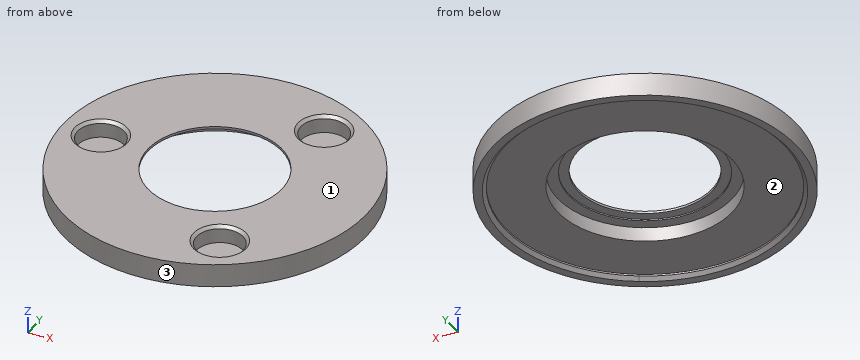
Autodesk Inventor part; units mm, degrees
ref_plane "YZ Plane" through (0, 0, 0) normal (1, 0, 0) x (0, 1, 0)
ref_plane "XZ Plane" through (0, 0, 0) normal (0, 1, 0) x (-1, 0, 0)
ref_plane "XY Plane" through (0, 0, 0) normal (0, 0, 1) x (1, 0, 0)
ref_plane "Arbeitsebene1" through (0, -18.5, -1.048) normal (1, 0, 0) x (0, 0, -1)
sketch "Skizze1" plane through (0, -18.5, -1.048) normal (1, 0, 0) x (0, 0, -1)
  line L0 (-1.65, 12.5) -> (-1.5, 12.5)
  line L1 (-1.5, -12.5) -> (-1.5, 12.5)
  line L2 (-1.65, 12.5) -> (-1.65, -12.5)
  line L3 (8.4324, 0) -> (-3.3304, 0)
  line L4 (-1.6429, 13.1) -> (-1.65, 13.1)
  line L5 (-1.65, 13.1) -> (-1.65, 11.5)
  line L6 (-1.65, 11.5) -> (-2.05, 11.5)
  line L7 (-2.05, 11.5) -> (-2.05, 23.9922)
  line L8 (-2.05, 23.9922) -> (1.05, 23.9922)
  line L9 (1.05, 23.9922) -> (1.05, 14.9922)
  line L10 (1.552, 13.5) -> (-1.048, 13.5) construction
  line L11 (-1.65, 13.1) -> (-1.4, 13.1)
  line L12 (-1.4, 13.1) -> (-1.4, 14.9922)
  line L13 (-1.4, 14.9922) -> (1.05, 14.9922)
  point P0 (-1.048, 18.5)
  dimension "d0" = 0.4
  dimension "d1" = 3.1
  dimension "d2" = 9
  dimension "d3" = 0.6
  dimension "d4" = 0
  dimension "d5" = 1
  dimension "d6" = 0.25
revolve "Umdrehung1" add sketch "Skizze1" angle 360 about axis through (0, -18.5, -9.4804) along (0, 0, 1) contours L2 L6 L7 L8 L9 L13 L12 L11 L4 L5
sketch "Skizze2" plane through (0, -18.5, 1.002) normal (0, 0, -1) x (-1, 0, 0)
  circle A0 centre (0, 0) radius 14.9922
  circle A1 centre (0, 0) radius 23.9922
  line L0 (19.4922, 0) -> (-9.7461, -16.8807) construction
  line L1 (-9.7461, -16.8807) -> (-9.7461, 16.8807) construction
  line L2 (-9.7461, 16.8807) -> (19.4922, 0) construction
  circle A2 centre (19.4922, 0) radius 4
  circle A3 centre (-9.7461, -16.8807) radius 4
  circle A4 centre (-9.7461, 16.8807) radius 4
  point P0 (0, 18.5)
  dimension "d8" = 47.9844
  dimension "d9" = 29.9844
  dimension "d10" = 19.4922
  dimension "d11" = 8
  dimension "d12" = 8
  dimension "d13" = 8
extrude "Extrusion1" cut sketch "Skizze2" along normal blind 3 contours A2 | A3 | A4
chamfer "Fase1" distance 0.5 angle 45 3 edges at (13.7461, -1.6193, 1.002) (13.7461, -35.3807, 1.002) (-15.4922, -18.5, 1.002)
sketch "Skizze3" plane through (0, -18.5, 1.002) normal (0, 0, 1) x (1, 0, 0)
  arc A0 (11.9961, -20.7778) -> (11.9961, 20.7778) centre (0, 0) ccw
  circle A1 centre (0, 0) radius 23.9922
  circle A2 centre (0, 0) radius 26
  point P0 (0, 18.5)
  point P1 (11.9961, -20.7778)
  point P2 (11.9961, 20.7778)
  dimension "d19" = 52
extrude "Extrusion2" add sketch "Skizze3" against normal blind 4
chamfer "Fase2" distance 0.6 angle 45 1 edges at (-11.9961, -39.2778, -2.998)
equation "\"d10\" = 0.25 * d9 + 0.25 * d8"
properties part number "02_SMLM_Holdre_Bottom"
CAD build for the part. Positions are in the model's coordinates, mm. Face numbers are marked on the shaded views. Round coordinates to 2 decimals unless told otherwise and drop trailing zeros. Loops run counter-clockwise (first coordinate to the right, second up) from the corner with the lowest first, then second, coordinate; pieces in that order, holes last.
(1) Cut at B-B (y = -18.5). Give the cut face in (x, z).
(2) Two-plate mould, pull along Y, no slides. Class the marked faces 1, 2 and 3: +Y half, -Y half, draft (parallel to the pull), parting line (faces both ways), or undercut.
(3) Wall check: line 1 along Y through (x, z) = (0, 0.8); line 2 along X through (y, z) = (-22, 0.65); line 3 along Y through (x, z) = (0, -2.2). Give the ranges that are in metal, low to high.
(4) Drop flat-ended pins along their axis: pin 1 (2.5 mm diameter, centred on x = -19.5, y = -19, fed in from +Z); pin 2 (7 mm diameter, centred on x = 9.75, y = -1.62, fed in from -Z); pin 3 (2 mm diameter, centred on y = -5.5, z = -2.5, fed in from -X). Give the stop position or say it passes through.
(5) Cut at A-A (z = -1.35). Give the cut face in (x, y), plus the area to 3 significant figures.
Findings below:
1. outline: (-26, -3) - (-24.59, -3) - (-23.99, -2.4) - (-23.99, -2.1) - (-14.99, -2.1) - (-14.99, 0.35) - (-13.1, 0.35) - (-13.1, 0.6) - (-11.5, 0.6) - (-11.5, 1) - (-14.99, 1) - (-15.49, 0.5) - (-15.49, -2) - (-23.49, -2) - (-23.49, 0.5) - (-23.99, 1) - (-26, 1) - close; (11.5, 0.6) - (13.1, 0.6) - (13.1, 0.35) - (14.99, 0.35) - (14.99, -2.1) - (23.99, -2.1) - (23.99, -2.4) - (24.59, -3) - (26, -3) - (26, 1) - (11.5, 1) - close
2. face 1: draft
2. face 2: undercut
2. face 3: parting line
3. line 1: y = -44.5 to -30, -7 to 7.5
3. line 2: x = -25.76 to -21.72, -17.27 to -10.95, 10.95 to 25.76
3. line 3: y = -44.5 to -42.49, 5.49 to 7.5
4. pin 1: stops at z = -2
4. pin 2: stops at z = -2.1
4. pin 3: stops at x = -23.07
5. outline: circle Ø52 at (0, -18.5); hole circle Ø8 at (-19.49, -18.5); hole circle Ø29.98 at (0, -18.5); hole circle Ø8 at (9.75, -35.38); hole circle Ø8 at (9.75, -1.62)
5. area: 1,270 mm2
